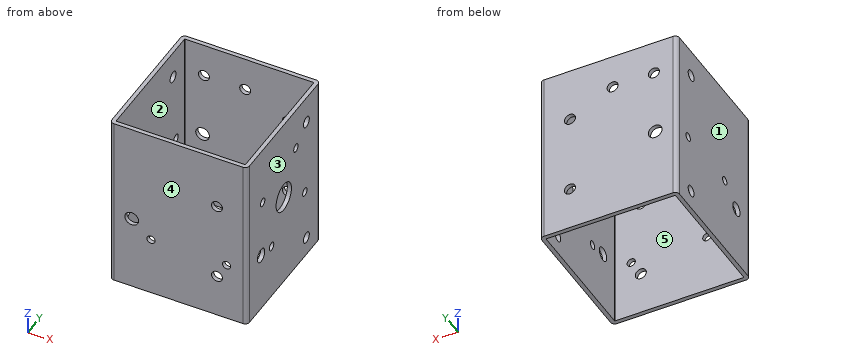
from build123d import *

# Parameters (mm, degrees)
SKETCH1_W                      = 100
SKETCH1_H                      = 100
SKETCH1_W_2                    = 94
SKETCH1_H_2                    = 94
EXTRUDE_THIN1_DEPTH            = 130
FILLET1_R                      = 0.5
FILLET2_R                      = 3
F_8_0_8_DIAMETER_HOLE2_D       = 8
F_8_0_8_DIAMETER_HOLE3_D       = 8
F_10_0_10_DIAMETER_HOLE1_D     = 10
F_10_0_10_DIAMETER_HOLE2_D     = 10
F_6_0_6_DIAMETER_HOLE2_D       = 6
F_6_0_6_DIAMETER_HOLE2_DEPTH   = 3
F_6_0_6_DIAMETER_HOLE3_D       = 6
F_6_0_6_DIAMETER_HOLE3_DEPTH   = 3
F_21_0_21_DIAMETER_HOLE1_D     = 21
F_21_0_21_DIAMETER_HOLE1_DEPTH = 3
F_6_0_6_DIAMETER_HOLE1_D       = 6
F_6_0_6_DIAMETER_HOLE1_DEPTH   = 3
F_8_0_8_DIAMETER_HOLE4_D       = 8
F_8_0_8_DIAMETER_HOLE4_DEPTH   = 3
SKETCH33_R                     = 4
CUT_EXTRUDE1_DEPTH             = 10


with BuildPart() as part:
    # Sketch1 → Extrude-Thin1 (new body)
    with BuildSketch(Plane.XY):
        Rectangle(SKETCH1_W, SKETCH1_H)
        Rectangle(SKETCH1_W_2, SKETCH1_H_2, mode=Mode.SUBTRACT)
    extrude(amount=EXTRUDE_THIN1_DEPTH)

    # Fillet1
    fillet1_edges = [part.edges().sort_by_distance(p)[0] for p in [
        (47, -47, 65),
        (47, 47, 65),
        (-47, 47, 65),
        (-47, -47, 65),
    ]]
    fillet(fillet1_edges, radius=FILLET1_R)

    # Fillet2
    fillet2_edges = [part.edges().sort_by_distance(p)[0] for p in [
        (50, -50, 65),
        (-50, -50, 65),
        (-50, 50, 65),
        (50, 50, 65),
    ]]
    fillet(fillet2_edges, radius=FILLET2_R)

    # Ø8.0 (8) Diameter Hole2 (through all)
    with Locations(Plane(origin=(0, 50, 0), x_dir=(1, 0, 0), z_dir=(0, 1, 0))):
        with Locations((28, -32), (28, -90)):
            Hole(F_8_0_8_DIAMETER_HOLE2_D / 2)

    # Ø8.0 (8) Diameter Hole3 (through all)
    with Locations(Plane(origin=(50, 0, 0), x_dir=(0, 0, -1), z_dir=(1, 0, 0))):
        with Locations((-14, 31), (-110, 31)):
            Hole(F_8_0_8_DIAMETER_HOLE3_D / 2)

    # Ø10.0 (10) Diameter Hole1 (through all)
    with Locations(Plane(origin=(0, 50, 0), x_dir=(1, 0, 0), z_dir=(0, 1, 0))):
        with Locations((-34, -56)):
            Hole(F_10_0_10_DIAMETER_HOLE1_D / 2)

    # Ø10.0 (10) Diameter Hole2 (through all)
    with Locations(Plane(origin=(50, 0, 0), x_dir=(0, 0, -1), z_dir=(1, 0, 0))):
        with Locations((-44, -31)):
            Hole(F_10_0_10_DIAMETER_HOLE2_D / 2)

    # Ø6.0 (6) Diameter Hole2
    with Locations(Plane.ZY.offset(50)):
        with Locations((56, -15), (56, 35)):
            Hole(F_6_0_6_DIAMETER_HOLE2_D / 2, depth=F_6_0_6_DIAMETER_HOLE2_DEPTH)

    # Ø6.0 (6) Diameter Hole3
    with Locations(Plane(origin=(0, -50, 0), x_dir=(-1, 0, 0), z_dir=(0, -1, 0))):
        with Locations((20, -44), (-35, -44)):
            Hole(F_6_0_6_DIAMETER_HOLE3_D / 2, depth=F_6_0_6_DIAMETER_HOLE3_DEPTH)

    # Ø21.0 (21) Diameter Hole1
    with Locations(Plane(origin=(50, 0, 0), x_dir=(0, 0, -1), z_dir=(1, 0, 0))):
        with Locations((-70, 0)):
            Hole(F_21_0_21_DIAMETER_HOLE1_D / 2, depth=F_21_0_21_DIAMETER_HOLE1_DEPTH)

    # Ø6.0 (6) Diameter Hole1
    with Locations(Plane(origin=(50, 0, 0), x_dir=(0, 0, -1), z_dir=(1, 0, 0))):
        with Locations((-41.157258279, -16.652364697), (-53.347635303, 28.842741721), (-98.842741721, 16.652364697), (-86.652364697, -28.842741721)):
            Hole(F_6_0_6_DIAMETER_HOLE1_D / 2, depth=F_6_0_6_DIAMETER_HOLE1_DEPTH)

    # Ø8.0 (8) Diameter Hole4
    with Locations(Plane(origin=(0, 50, 0), x_dir=(1, 0, 0), z_dir=(0, 1, 0))):
        with Locations((-3, -105)):
            Hole(F_8_0_8_DIAMETER_HOLE4_D / 2, depth=F_8_0_8_DIAMETER_HOLE4_DEPTH)

    # Sketch33 → Cut-Extrude1 (cut)
    with BuildSketch(Plane(origin=(0, 50, 0), x_dir=(1, 0, 0), z_dir=(0, 1, 0))):
        with Locations(Location((-33, -105, 0), (0, 0, 270))):
            Circle(SKETCH33_R)
    extrude(amount=-CUT_EXTRUDE1_DEPTH, mode=Mode.SUBTRACT)


solid = part.part
The listing builds one solid part. Answer for the finished solid, in the listing's coordinates (mm). Face numbers are marked on the shaded views. A direction names the side the tool comes from. Give positions to 0.01 mm unless a question says otherwise; leave off trailing zeros. Loops run counter-clockwise (first coordinate to the right, second up) from the corner with the lowest first, then second, coordinate; pieces in that order, holes last. Notation, with made-up numbers: (75.25, 58) - (129.25, 58) arc R16 ccw to (129.25, 85) - close; hole circle Ø1 at (76.5, 5). An arc over 180 degrees is marked (long way). Answer as a JSON object with one key per item and string values.
1. A cutting plane is placed at C-C (x = 14.5). Write down the section's boundary in (y, z), then the cut area to 3 significant figures.
Determined:
{"outline": "(-50, 0) - (-47, 0) - (-47, 130) - (-50, 130) - close; (47, 0) - (50, 0) - (50, 130) - (47, 130) - close", "area": "780 mm²"}
2. Find the intervals of material crossed by L1, parallel to X at y = -20, z = 11; L2, parallel to Z at x = 35, y = -48.8, in increasing order. Write a range as [from, to].
Determined:
{"L1": "[-50, -47], [47, 50]", "L2": "[0, 41], [47, 130]"}
3. A cutting plane is placed at B-B (x = -3). Write down the section's boundary in (y, z).
Determined:
{"outline": "(-50, 0) - (-47, 0) - (-47, 130) - (-50, 130) - close; (47, 0) - (50, 0) - (50, 101) - (47, 101) - close; (47, 109) - (50, 109) - (50, 130) - (47, 130) - close"}
4. A cutting plane is placed at A-A (z = 14). Write down the section's boundary in (x, y), then the cut area to 3 significant figures.
Determined:
{"outline": "(-50, -47) arc R3 ccw to (-47, -50) - (47, -50) arc R3 ccw to (50, -47) - (50, 27) - (47, 27) - (47, -46.5) arc R0.5 cw to (46.5, -47) - (-46.5, -47) arc R0.5 cw to (-47, -46.5) - (-47, 27) - (-50, 27) - close; (-50, 35) - (-47, 35) - (-47, 46.5) arc R0.5 cw to (-46.5, 47) - (46.5, 47) arc R0.5 cw to (47, 46.5) - (47, 35) - (50, 35) - (50, 47) arc R3 ccw to (47, 50) - (-47, 50) arc R3 ccw to (-50, 47) - close", "area": "1,110 mm²"}
5. Flat-ended cylindrical pins translate along their axes: pin 1 Ø13 at (x, z) = (-34, 56) entering from -Y; pin 2 Ø5 at (x, z) = (-3, 105) entering from +Y; pin 3 Ø3.5 at (y, z) = (-15, 56) entering from -X. Find the tip coordinate at first contact, or state that the pin passes through.
Determined:
{"pin 1": "y = -50", "pin 2": "y = -47", "pin 3": "x = 47"}
6. For the marked faces 4 and 5, determine the directions among +Z, -Z, +X, -X, +Y, -Y from which every point of the face is accessible in a straight line to the end or side of a thin tool.
Determined:
{"face 4": "+Z, -Z, +X, -X, -Y", "face 5": "+Z, -Z"}
7. A cutting plane is placed at D-D (y = -2). Write down the section's boundary in (x, z).
Determined:
{"outline": "(-50, 0) - (-47, 0) - (-47, 130) - (-50, 130) - close; (47, 0) - (50, 0) - (50, 59.69) - (47, 59.69) - close; (47, 80.31) - (50, 80.31) - (50, 130) - (47, 130) - close"}
8. For a pull along X with two mould halves and no side action, classify the marked faces 1, 2 and 3 as pulls with the +X half, pulls with the -X half, needs draft (parallel to the pull), parting line crosses it, or undercut.
Determined:
{"face 1": "pulls with the -X half", "face 2": "undercut", "face 3": "pulls with the +X half"}
